```python
from build123d import *

# Parameters (mm, degrees)
F0_R     = 18.5
F0_R_2   = 5
F1_DEPTH = 1.3
F2_DEPTH = 4.6
F0_W     = 15
F0_H     = 3
F0_H_2   = 5.176528
F0_W_2   = 2.5
F0_H_3   = 15
F0_W_3   = 5
F3_DEPTH = 4.6
F4_DEPTH = 12
F5_DEPTH = 9
F6_R     = 5


with BuildPart() as f1:
    # F0 (on Top) → F1 (new body)
    with BuildSketch(Plane.XY):
        with BuildLine():
            ThreePointArc((20.149442, -7.5), (21.159667, -3.810315), (21.5, 0))
            ThreePointArc((21.5, 0), (21.159667, 3.810315), (20.149442, 7.5))
            ThreePointArc((20.149442, 7.5), (15.202796, 15.202796), (7.5, 20.149442))
            ThreePointArc((7.5, 20.149442), (0, 21.5), (-7.5, 20.149442))
            ThreePointArc((-7.5, 20.149442), (-15.202796, 15.202796), (-20.149442, 7.5))
            ThreePointArc((-20.149442, 7.5), (-21.5, 0), (-20.149442, -7.5))
            ThreePointArc((-20.149442, -7.5), (0, -21.5), (20.149442, -7.5))
        make_face()
        Circle(F0_R, mode=Mode.SUBTRACT)
        Circle(F0_R)
        Circle(F0_R_2, mode=Mode.SUBTRACT)
    extrude(amount=F1_DEPTH)

    # F0 (on Top) → F2 (join)
    with BuildSketch(Plane.XY):
        with BuildLine():
            ThreePointArc((20.149442, -7.5), (21.159667, -3.810315), (21.5, 0))
            ThreePointArc((21.5, 0), (21.159667, 3.810315), (20.149442, 7.5))
            ThreePointArc((20.149442, 7.5), (15.202796, 15.202796), (7.5, 20.149442))
            ThreePointArc((7.5, 20.149442), (0, 21.5), (-7.5, 20.149442))
            ThreePointArc((-7.5, 20.149442), (-15.202796, 15.202796), (-20.149442, 7.5))
            ThreePointArc((-20.149442, 7.5), (-21.5, 0), (-20.149442, -7.5))
            ThreePointArc((-20.149442, -7.5), (0, -21.5), (20.149442, -7.5))
        make_face()
        Circle(F0_R, mode=Mode.SUBTRACT)
    extrude(amount=F2_DEPTH)

    # F0 (on Top) → F3 (join)
    with BuildSketch(Plane.XY):
        with Locations((0, 38.507013)):
            Rectangle(F0_W, F0_H)
        with Locations((0, 34.418749)):
            Rectangle(F0_W, F0_H_2)
        with BuildLine():
            ThreePointArc((-7.5, 20.149442), (0, 21.5), (7.5, 20.149442))
            Line((7.5, 20.149442), (7.5, 31.830485))
            Line((7.5, 31.830485), (-7.5, 31.830485))
            Line((-7.5, 31.830485), (-7.5, 20.149442))
        make_face()
        with Locations((-38.75, 0)):
            Rectangle(F0_W_2, F0_H_3)
        with Locations((-35, 0)):
            Rectangle(F0_W_3, F0_H_3)
        with BuildLine():
            Line((-32.5, -7.5), (-20.149442, -7.5))
            ThreePointArc((-20.149442, -7.5), (-21.5, 0), (-20.149442, 7.5))
            Line((-20.149442, 7.5), (-32.5, 7.5))
            Line((-32.5, 7.5), (-32.5, -7.5))
        make_face()
        with BuildLine():
            ThreePointArc((20.149442, 7.5), (21.159667, 3.810315), (21.5, 0))
            ThreePointArc((21.5, 0), (21.159667, -3.810315), (20.149442, -7.5))
            Line((20.149442, -7.5), (32.5, -7.5))
            Line((32.5, -7.5), (32.5, 7.5))
            Line((32.5, 7.5), (20.149442, 7.5))
        make_face()
        with Locations((35, 0)):
            Rectangle(F0_W_3, F0_H_3)
        with Locations((38.75, 0)):
            Rectangle(F0_W_2, F0_H_3)
    extrude(amount=F3_DEPTH)

    # F0 (on Top) → F4 (join)
    with BuildSketch(Plane.XY):
        with Locations((0, 34.418749)):
            Rectangle(F0_W, F0_H_2)
        with Locations((0, 38.507013)):
            Rectangle(F0_W, F0_H)
        with Locations((38.75, 0)):
            Rectangle(F0_W_2, F0_H_3)
        with Locations((35, 0)):
            Rectangle(F0_W_3, F0_H_3)
        with Locations((-35, 0)):
            Rectangle(F0_W_3, F0_H_3)
        with Locations((-38.75, 0)):
            Rectangle(F0_W_2, F0_H_3)
    extrude(amount=-F4_DEPTH)

    # F0 (on Top) → F5 (cut)
    with BuildSketch(Plane.XY):
        with Locations((35, 0)):
            Rectangle(F0_W_3, F0_H_3)
        with Locations((-35, 0)):
            Rectangle(F0_W_3, F0_H_3)
        with Locations((0, 34.418749)):
            Rectangle(F0_W, F0_H_2)
    extrude(amount=-F5_DEPTH, mode=Mode.SUBTRACT)

    # F6
    f6_edges = [f1.edges().sort_by_distance(p)[0] for p in [
        (7.5, 20.149442, 2.3),
        (20.149442, -7.5, 2.3),
        (20.149442, 7.5, 2.3),
        (-7.5, 20.149442, 2.3),
        (-20.149442, 7.5, 2.3),
        (-20.149442, -7.5, 2.3),
    ]]
    fillet(f6_edges, radius=F6_R)


solid = f1.part
```
Here's how the part is built. I have some questions about the finished solid (model axes, mm). A direction names the side the tool comes from. Give positions to 0.01 mm unless a question says otherwise; leave off trailing zeros. Write each loop counter-clockwise with the first axis right and the second up, starting at its lowest first coordinate (ties: lowest second). Pieces come first, ordered by that corner, then holes. Notation, with made-up numbers: M 65,-25 L 84,-25 A21 ccw 84,10 Z; hole C 28,19 d8. An arc over 180 degrees is marked long. Put each result on its own line as item: value. Start each with the question number.
Item 1: Thinking about a two-plate mould opening in Z: for faces 1 (the flat face through (0, 36, -12)), 2 (the cylindrical face through (8.23, 20.765, 2.332)), 3 (the flat face through (37.5, 0, -4)), which applies, +Z half, -Z half, draft (parallel to the pull), parting line (faces both ways), or undercut?
Item 2: Will these pins go through, and if not, where does the flat tip stop? pin 1 (12 mm diameter, centred on x = 15, y = -10.5, fed in from -Z); pin 2 (6 mm diameter, centred on y = 26.5, z = 1.5, fed in from -X); pin 3 (8 mm diameter, centred on x = 0, y = 0, fed in from +Z); pin 4 (5 mm diameter, centred on y = 33.5, z = 0.5, fed in from +X).
Item 3: If we section it at C-C, the plane x = 0: Write out the boundary of the cut face in (y, z), then the cut area to 3 significant figures.
Item 4: If we section it at B-B, the plane y = 0: Write out the boundary of the cut face in (x, z), then the cut area to 3 significant figures.
Item 5: If we section it at D-D, the plane y = 13.5: Write out the boundary of the cut face in (x, z), then the cut area to 3 significant figures.
Item 6: On a 3-axis mill with a long thin cutter (end or side, diameter ignored), from which of +Z, -Z, +X, -X, +Y, -Y can I reach the whole of each face in a straight line? I mean faces 4 (the flat face through (-7.5, 34, 2)), 5 (the flat face through (7.5, 33, 2)), 6 (the flat face through (0, 31.83, -10)), 7 (the flat face through (-34, -7.5, 2)). Say none if no direction works.
Item 7: I need wall thicknesses on L1, parallel to X at y = -3, z = -7.5; L2, parallel to X at y = 0, z = 3.5; L3, parallel to Z at x = -35.5, y = -3. Which ranges of each line are inside material? Lowest first, please. Write a range as from..to.
Item 8: If we section it at A-A, the plane z = -3: Write out the boundary of the cut face in (x, y).
Values:
1. face 1: -Z half
1. face 2: draft
1. face 3: undercut
2. pin 1: z = 0
2. pin 2: x = -7.5
2. pin 3: through
2. pin 4: x = 7.5
3. outline: M -21.5,0 L -5,0 L -5,1.3 L -18.5,1.3 L -18.5,4.6 L -21.5,4.6 Z; M 5,0 L 37.01,0 L 37.01,-9 L 31.83,-9 L 31.83,-12 L 40.01,-12 L 40.01,4.6 L 18.5,4.6 L 18.5,1.3 L 5,1.3 Z
3. area: 199 mm²
4. outline: M -40,-12 L -32.5,-12 L -32.5,-9 L -37.5,-9 L -37.5,0 L -5,0 L -5,1.3 L -18.5,1.3 L -18.5,4.6 L -40,4.6 Z; M 5,0 L 37.5,0 L 37.5,-9 L 32.5,-9 L 32.5,-12 L 40,-12 L 40,4.6 L 18.5,4.6 L 18.5,1.3 L 5,1.3 Z
4. area: 323 mm²
5. outline: M -16.73,0 L 16.73,0 L 16.73,4.6 L 12.65,4.6 L 12.65,1.3 L -12.65,1.3 L -12.65,4.6 L -16.73,4.6 Z
5. area: 70.5 mm²
6. face 4: +Z, -Z, -X, +Y
6. face 5: +Z, -Z, +X, +Y
6. face 6: -Z, +X, -X, -Y
6. face 7: +Z, -Z, -X, -Y
7. L1: -40..-37.5, 37.5..40
7. L2: -40..-18.5, 18.5..40
7. L3: -12..-9, 0..4.6
8. outline: M -40,-7.5 L -37.5,-7.5 L -37.5,7.5 L -40,7.5 Z; M -7.5,37.01 L 7.5,37.01 L 7.5,40.01 L -7.5,40.01 Z; M 37.5,-7.5 L 40,-7.5 L 40,7.5 L 37.5,7.5 Z
